from build123d import *

# Parameters (mm, degrees)
SKETCH1_R                 = 1
BOSS_EXTRUDE_9_10MM_DEPTH = 9.1
F_0_5_X_45_DEG_SIZE       = 0.5


with BuildPart() as part:
    # Sketch1 → Boss-Extrude 9.10mm (new body)
    with BuildSketch(Plane(origin=(0, 0, 0), x_dir=(1, 0, 0), z_dir=(0, 1, 0))):
        Circle(SKETCH1_R)
    extrude(amount=-BOSS_EXTRUDE_9_10MM_DEPTH)

    # 0.5 x 45 deg
    f_0_5_x_45_deg_edges = [part.edges().sort_by_distance(p)[0] for p in [
        (-1, -9.1, 0),
    ]]
    chamfer(f_0_5_x_45_deg_edges, length=F_0_5_X_45_DEG_SIZE)

    # Sketch2 → SR8 (revolve, cut)
    with BuildSketch(Plane.XY):
        with BuildLine():
            Line((0, 2), (-2, 2))
            Line((-2, 2), (-2, -0.254033308))
            ThreePointArc((-2, -0.254033308), (-1.00803434, -0.06376243), (0, 0))
            Line((0, 0), (0, 2))
        make_face()
    revolve(axis=Axis((0, 0, 0), (0, 1, 0)), mode=Mode.SUBTRACT)


solid = part.part
Read the model definition and answer for the solid it produces. Units are mm, in the model's axes. Round coordinates to 2 decimals unless told otherwise and drop trailing zeros. Write each loop counter-clockwise with the first axis right and the second up, starting at its lowest first coordinate (ties: lowest second). Pieces come first, ordered by that corner, then holes.
1. Straight lines are drawn through the part: L1, parallel to Z at x = -0.05, y = -3.75; L2, parallel to Y at x = 0.6, z = -0.1. For each, find the intervals that lie inside material, in ascending order.
2. The part is cut by section B-B, the plane z = 0. Determine the outline of the cut face in (x, y), then the cut area to 3 significant figures.
3. The part is cut by section C-C, the plane y = -2.25. Determine the outline of the cut face in (x, z).
4. The part is cut by section A-A, the plane x = 0. Determine the outline of the cut face in (y, z).
Values:
1. L1: z = -1 to 1
1. L2: y = -8.99 to -0.02
2. outline: (-1, -8.6) - (-0.5, -9.1) - (0.5, -9.1) - (1, -8.6) - (1, -0.06) arc R8 ccw to (-1, -0.06) - close
2. area: 17.9 mm2
3. outline: circle Ø2 at (0, 0)
4. outline: (-9.1, -0.5) - (-8.6, -1) - (-0.06, -1) arc R8 ccw to (-0.06, 1) - (-8.6, 1) - (-9.1, 0.5) - close
